Here's how the part is built. I have some questions about the finished solid (model axes, mm). A direction names the side the tool comes from. Coordinates: 2 decimals unless noted, no trailing zeros. Answer in a Markdown table with one row per item. Add a question column.
Item 1: Imagine slicing it at A-A (y = -4.5). State how many separate pieces and enclosed holes the cut face has, plus the area to 3 significant figures.
Item 2: Which directions (+Z, -Z, +X, -X, +Y, -Y) give clear straight access to the entire face, cutting with the end or side of a thin tool? Please do faces 1 (the face through (2.244, -7, 5)), 2 (the face through (-60, -1, 5)).
Item 3: We'd pull the mould along X, two halves only. Please class faces 3 (the face through (1, 1, 10)), 4 (the face through (16, -15.833, 5)), 5 (the face through (57.15, -56.99, 4.93)): +X half, -X half, draft (parallel to the pull), parting line (faces both ways), or undercut.
Item 4: If I drill on probe 1 along Y at (x, z) = (-24, 8); probe 2 along X at (y, z) = (-15.5, 5.25); probe 3 along Y at (x, z) = (-15, 4), over which ranges is the centre line in solid material (lowest first)? Write a range as from..to.
from build123d import *

# Parameters (mm, degrees)
BOSS_EXTRUDE1_DEPTH = 10
CUT_EXTRUDE20_DEPTH = 10


with BuildPart() as part:
    # Sketch1 → Boss-Extrude1 (new body)
    with BuildSketch(Plane.XY):
        with BuildLine():
            Line((-50, 60), (50, 60))
            ThreePointArc((50, 60), (57.071067812, 57.071067812), (60, 50))
            Line((60, 50), (60, -50))
            ThreePointArc((60, -50), (57.071067812, -57.071067812), (50, -60))
            Line((50, -60), (-50, -60))
            ThreePointArc((-50, -60), (-57.071067812, -57.071067812), (-60, -50))
            Line((-60, -50), (-60, 50))
            ThreePointArc((-60, 50), (-57.071067812, 57.071067812), (-50, 60))
        make_face()
    extrude(amount=BOSS_EXTRUDE1_DEPTH)

    # Sketch2 → Cut-Extrude20 (cut)
    with BuildSketch(Plane.XY.offset(10)):
        with BuildLine():
            Line((43.025841346, 32.389823718), (30.123197115, 20.0390625))
            add(Edge.make_bspline(
                [(30.123197115, 20.0390625), (29.101672257, 21.061811325), (27.097271839, 23.068613369), (23.819325693, 25.680604146), (20.424368315, 27.901312672), (16.901225536, 29.727334557), (13.244989599, 31.143755892), (9.462875821, 32.156967391), (5.548731191, 32.7579203), (2.899029992, 32.842051661), (1.55849359, 32.884615385)],
                knots=[0, 0, 0, 0, 1.075575784, 2.110457258, 3.113929901, 4.09197124, 5.059417775, 6.02750972, 7.002078037, 8, 8, 8, 8], degree=3))
            add(Edge.make_bspline(
                [(1.55849359, 32.884615385), (0.396289515, 32.854791176), (-1.885800065, 32.796228727), (-5.239110912, 32.351509499), (-8.443404835, 31.608626028), (-11.513820243, 30.579485021), (-14.431611188, 29.240247299), (-17.213683889, 27.611582431), (-19.842917451, 25.681030991), (-22.298608552, 23.485189523), (-24.534523201, 21.087773984), (-26.486594752, 18.521691616), (-28.149340344, 15.834772023), (-29.518119077, 13.01326852), (-30.559610844, 10.06151156), (-31.303099679, 6.981643968), (-31.775030209, 3.782616261), (-31.830751107, 1.600206429), (-31.858974359, 0.494791667)],
                knots=[0, 0, 0, 0, 1.075001177, 2.110859044, 3.123021556, 4.114053297, 5.101481495, 6.087880186, 7.091499647, 8.114004866, 9.131394192, 10.11971144, 11.092043119, 12.050101265, 13.015322563, 13.981809771, 14.977764287, 16, 16, 16, 16], degree=3))
            add(Edge.make_bspline(
                [(-31.858974359, 0.494791667), (-31.83264906, -0.648882984), (-31.780784616, -2.90207861), (-31.282567998, -6.208740054), (-30.514979525, -9.389986642), (-29.39143466, -12.422214259), (-28.0086912, -15.346960195), (-26.255144671, -18.107569332), (-24.210333942, -20.746199204), (-21.877912803, -23.216909745), (-19.340840935, -25.494310256), (-16.593109559, -27.458854559), (-13.718321506, -29.153832231), (-10.670077564, -30.496199757), (-7.501286227, -31.573973822), (-4.179806851, -32.333897032), (-0.713118606, -32.800107284), (1.652171532, -32.856165602), (2.852564103, -32.884615385)],
                knots=[0, 0, 0, 0, 1.022067601, 2.013613092, 2.983553406, 3.943623673, 4.90013463, 5.87121881, 6.861774014, 7.881098904, 8.905697761, 9.905387765, 10.89678721, 11.884561068, 12.87834324, 13.885584958, 14.926927371, 16, 16, 16, 16], degree=3))
            add(Edge.make_bspline(
                [(2.852564103, -32.884615385), (3.633375016, -32.877570263), (5.166280575, -32.863739121), (7.414791803, -32.639220794), (9.56832549, -32.318245747), (11.635221676, -31.893312898), (13.594610257, -31.291956666), (15.47362031, -30.588744605), (17.261242491, -29.758814157), (18.947784497, -28.773531178), (20.558346969, -27.669149395), (22.077854726, -26.405501787), (23.532961722, -25.011078956), (24.906665222, -23.468846061), (26.175714886, -21.765013702), (27.380767856, -19.930892086), (28.508026478, -17.948278664), (29.174093857, -16.548257493), (29.514222756, -15.833333333)],
                knots=[0, 0, 0, 0, 1.109579412, 2.178351274, 3.208885622, 4.204702371, 5.174744997, 6.119429583, 7.05542196, 7.97267548, 8.893247984, 9.828544973, 10.778894627, 11.756245826, 12.760884819, 13.796418446, 14.874735809, 16, 16, 16, 16], degree=3))
            Line((29.514222756, -15.833333333), (2.243589744, -15.833333333))
            Line((2.243589744, -15.833333333), (2.243589744, 1.217948718))
            Line((2.243589744, 1.217948718), (49.610376603, 1.217948718))
            Line((49.610376603, 1.217948718), (49.743589744, -2.835536859))
            add(Edge.make_bspline(
                [(49.743589744, -2.835536859), (49.726472847, -3.876574804), (49.692269599, -5.95679287), (49.379687785, -9.05388319), (48.861900774, -12.109897034), (48.154036366, -15.12176501), (47.266903196, -18.104261414), (46.135530703, -21.028826361), (44.810700427, -23.915293277), (43.326322097, -26.751396909), (41.658307942, -29.472715457), (39.862445782, -32.049444886), (37.964336859, -34.477125435), (35.922698088, -36.721933428), (33.769321141, -38.80272625), (31.499967076, -40.711498835), (29.106609302, -42.449866244), (26.601926388, -44.03251371), (23.971651757, -45.419610834), (21.230246649, -46.626201315), (18.381850215, -47.650933134), (15.419108562, -48.490990308), (12.347851627, -49.139161247), (9.168013616, -49.583612912), (5.877848125, -49.885622812), (3.646198469, -49.91893663), (2.510016026, -49.935897436)],
                knots=[0, 0, 0, 0, 1.006889344, 2.011981806, 3.007738725, 4.003571281, 5.003404394, 6.015442001, 7.03424805, 8.074616296, 9.110249922, 10.119753985, 11.111721717, 12.089233633, 13.052717867, 14.006597561, 14.955430184, 15.912305663, 16.870361111, 17.829300583, 18.807640451, 19.796414044, 20.806216501, 21.841577364, 22.90109906, 24, 24, 24, 24], degree=3))
            add(Edge.make_bspline(
                [(2.510016026, -49.935897436), (1.297786391, -49.919148326), (-1.105214309, -49.885946594), (-4.658372904, -49.574989776), (-8.108452155, -49.061775621), (-11.456312597, -48.351504768), (-14.709727285, -47.467515954), (-17.863106347, -46.357900887), (-20.910000278, -45.037978679), (-23.85953309, -43.54270137), (-26.674006547, -41.846926658), (-29.347112957, -39.980390143), (-31.864262001, -37.931085264), (-34.251237083, -35.733317811), (-36.452269248, -33.333066461), (-38.549382353, -30.808135004), (-40.44097845, -28.065919025), (-42.208390563, -25.195321967), (-43.778573599, -22.19754677), (-45.151721242, -19.128038823), (-46.322740771, -16.004570602), (-47.246117975, -12.812598182), (-47.995813786, -9.574378679), (-48.532235209, -6.275829811), (-48.83517745, -2.917364496), (-48.885118988, -0.660301834), (-48.91025641, 0.475761218)],
                knots=[0, 0, 0, 0, 1.084149091, 2.14910686, 3.187506334, 4.202448172, 5.208724393, 6.201130722, 7.189831603, 8.176984443, 9.156919086, 10.126598231, 11.090766514, 12.05840148, 13.026036446, 14.001772938, 14.991905635, 16.003017641, 17.015720547, 18.016462227, 19.009322657, 19.99686681, 20.986544154, 21.980959929, 22.983742515, 24, 24, 24, 24], degree=3))
            add(Edge.make_bspline(
                [(-48.91025641, 0.475761218), (-48.876592035, 2.025593992), (-48.810114873, 5.086054225), (-48.194435478, 9.594131562), (-47.234683024, 13.955246578), (-45.857341624, 18.15351638), (-44.089887361, 22.194724133), (-41.957357822, 26.088356769), (-39.413429836, 29.830275694), (-37.444254854, 32.14704321), (-36.4453125, 33.322315705)],
                knots=[0, 0, 0, 0, 1.034044851, 2.041932006, 3.031217818, 4.011390712, 4.986069675, 5.97149666, 6.970960976, 8, 8, 8, 8], degree=3))
            add(Edge.make_bspline(
                [(-36.4453125, 33.322315705), (-35.825078952, 34.002246466), (-34.593924689, 35.351898801), (-32.625926838, 37.227268178), (-30.608020011, 38.990184776), (-28.512255874, 40.603267051), (-26.349651476, 42.101826149), (-24.113982457, 43.457770387), (-21.816976621, 44.714273743), (-19.440720102, 45.807174398), (-16.997652934, 46.787051002), (-14.476955156, 47.616164385), (-11.897506276, 48.350561775), (-9.236465188, 48.909249832), (-6.520714756, 49.374482609), (-3.730977675, 49.686305981), (-0.874856146, 49.914850314), (1.056880807, 49.928826235), (2.034254808, 49.935897436)],
                knots=[0, 0, 0, 0, 1.020590567, 2.025856924, 3.013483481, 3.991664875, 4.957826714, 5.930500614, 6.890802512, 7.860442893, 8.829981142, 9.809047939, 10.802672283, 11.803273349, 12.823572789, 13.857849586, 14.916166035, 16, 16, 16, 16], degree=3))
            add(Edge.make_bspline(
                [(2.034254808, 49.935897436), (3.055927959, 49.920141479), (5.088682381, 49.888792909), (8.111051578, 49.671881266), (11.091422928, 49.337237729), (14.017236856, 48.835253312), (16.898312407, 48.216202044), (19.719736444, 47.423044151), (22.499915266, 46.521873915), (24.309801151, 45.803394427), (25.213341346, 45.444711538)],
                knots=[0, 0, 0, 0, 1.03180557, 2.052914215, 3.058998889, 4.059601663, 5.049854447, 6.033765722, 7.018406786, 8, 8, 8, 8], degree=3))
            add(Edge.make_bspline(
                [(25.213341346, 45.444711538), (25.973558652, 45.113223986), (27.519819621, 44.438987476), (29.769438752, 43.205440158), (32.024554321, 41.837911379), (34.260832481, 40.286401114), (36.474865772, 38.553811407), (38.689771056, 36.667508217), (40.882937788, 34.60549617), (42.302289454, 33.137946044), (43.025841346, 32.389823718)],
                knots=[0, 0, 0, 0, 0.894392155, 1.819168899, 2.76525314, 3.739198753, 4.75366411, 5.797420238, 6.877176959, 8, 8, 8, 8], degree=3))
        make_face()
    extrude(amount=-CUT_EXTRUDE20_DEPTH, mode=Mode.SUBTRACT)


solid = part.part
Here are the results:
| question | item | result |
|---|---|---|
| 1 | separate pieces | 3 |
| 1 | enclosed holes | 0 |
| 1 | area | 554 mm2 |
| 2 | face 1 | +Z, -Z |
| 2 | face 2 | +Z, -Z, -X, +Y, -Y |
| 3 | face 3 | draft |
| 3 | face 4 | undercut |
| 3 | face 5 | +X half |
| 4 | probe 1 | y = -60..-43.42, -20.91..21.62, 43.5..60 |
| 4 | probe 2 | x = -60..-46.44, -27.85..2.24, 48.02..60 |
| 4 | probe 3 | y = -60..-47.33, -28.38..28.88, 47.43..60 |
